Verification items for the finished model (mm, model axes). Face numbers are marked on the shaded views. A direction names the side the tool comes from. Coordinates: 2 decimals unless noted, no trailing zeros. Order: outer loops, then holes, each group sorted by start corner. A loop starts at its lowest first (then second) coordinate and runs counter-clockwise, first axis right, second up. Notation, with made-up numbers: (-24, 21) -> (8, 21) arc R18 cw to (8, 46) -> close; hole circle Ø10 at (0.5, 63.5). An arc over 180 degrees is marked (long way). Use CSV: the item, a comma, the result in double quotes. Start each with the question number.
1) Tool access check on the marked faces 1, 2 and 3. Record the directions out of +Z, -Z, +X, -X, +Y, -Y that give a thin tool (end or side, any length) a straight path to the whole face; none if there is none.
2) Go/stop test with flat-tipped pins: pin 1 (8.5 mm diameter, centred on x = 0, y = -8, fed in from +Z); pin 2 (8.5 mm diameter, centred on x = 0, y = -8, fed in from -Z); pin 3 (2.5 mm diameter, centred on x = 11.5, z = 1, fed in from +Y); pin 4 (5.5 mm diameter, centred on x = 11.25, y = -5.25, fed in from -Z). Record where each tip stops, or that it passes through.
3) Scan lines: line 1 along Y through (x, z) = (1.5, 1.6) (3 decimals); line 2 along Y through (x, z) = (0, 4.2); line 3 along X through (y, z) = (6.5, 3.7). Record each from-to range of solid material in increasing order.
4) Sectioned sample at D-D on y = -7.5. Record the boundary of the cut face in (x, z), then the cut area to 3 significant figures.
5) Sectioned sample at A-A on x = 0. Record the boundary of the cut face in (y, z), then the cut area to 3 significant figures.
6) Sectioned sample at B-B on x = -11.25. Record the boundary of the cut face in (y, z), then the cut area to 3 significant figures.
7) Release check for a two-part mould opening along Y. For the marked faces 4, 5 and 6 record: released by +Y, released by -Y, zero draft, split by the parting line, or undercut.
8) Sectioned sample at C-C on z = 3.8. Give the number of separate pieces and of enclosed holes in the cut face, then the cut area to 3 significant figures.
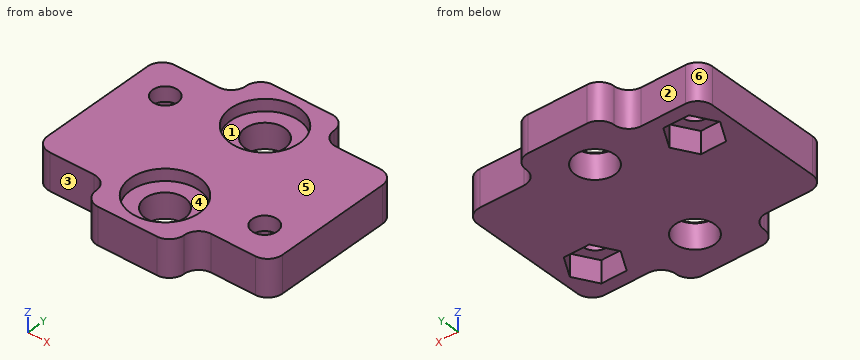
from build123d import *

# Parameters (mm, degrees)
SCHIZZO1_W                   = 32
SCHIZZO1_H                   = 20
ESTRUSIONE_ESTRUSIONE1_DEPTH = 5
SCHIZZO2_R                   = 1.7
TAGLIO_ESTRUSIONE1_DEPTH     = 20.519221296
SCHIZZO3_W                   = 12
SCHIZZO3_H                   = 4
ESTRUSIONE_ESTRUSIONE2_DEPTH = 5
SCHIZZO4_R                   = 4.7
TAGLIO_ESTRUSIONE2_DEPTH     = 1.6
SCHIZZO5_R                   = 2.7
TAGLIO_ESTRUSIONE3_DEPTH     = 22.530443563
TAGLIO_ESTRUSIONE4_DEPTH     = 3
RACCORDO1_R                  = 2


with BuildPart() as part:
    # Schizzo1 → Estrusione-Estrusione1 (new body)
    with BuildSketch(Plane.XY):
        Rectangle(SCHIZZO1_W, SCHIZZO1_H)
    extrude(amount=ESTRUSIONE_ESTRUSIONE1_DEPTH)

    # Schizzo2 → Taglio-Estrusione1 (cut, through all)
    with BuildSketch(Plane.XY.offset(5)):
        with Locations((-11.25, 5.25)):
            Circle(SCHIZZO2_R)
        with Locations((11.25, -5.25)):
            Circle(SCHIZZO2_R)
    extrude(amount=-TAGLIO_ESTRUSIONE1_DEPTH, mode=Mode.SUBTRACT)

    # Schizzo3 → Estrusione-Estrusione2 (add)
    with BuildSketch(Plane.XY):
        with Locations((0, 12)):
            Rectangle(SCHIZZO3_W, SCHIZZO3_H)
        with Locations((0, -12)):
            Rectangle(SCHIZZO3_W, SCHIZZO3_H)
    extrude(amount=ESTRUSIONE_ESTRUSIONE2_DEPTH)

    # Schizzo4 → Taglio-Estrusione2 (cut)
    with BuildSketch(Plane.XY.offset(5)):
        with Locations((0, 8)):
            Circle(SCHIZZO4_R)
        with Locations(Location((0, -8, 0), (0, 0, 180))):
            Circle(SCHIZZO4_R)
    extrude(amount=-TAGLIO_ESTRUSIONE2_DEPTH, mode=Mode.SUBTRACT)

    # Schizzo5 → Taglio-Estrusione3 (cut, through all)
    with BuildSketch(Plane.XY.offset(3.4)):
        with Locations((0, 8)):
            Circle(SCHIZZO5_R)
        with Locations((0, -8)):
            Circle(SCHIZZO5_R)
    extrude(amount=-TAGLIO_ESTRUSIONE3_DEPTH, mode=Mode.SUBTRACT)

    # Schizzo6 → Taglio-Estrusione4 (cut)
    with BuildSketch(Plane(origin=(0, 0, 0), x_dir=(-1, 0, 0), z_dir=(0, 0, -1))):
        Polygon((7.785898385, 5.25), (9.517949192, 2.25), (12.982050808, 2.25), (14.714101615, 5.25), (12.982050808, 8.25), (9.517949192, 8.25), align=None)
        Polygon((-14.714101615, -5.25), (-12.982050808, -8.25), (-9.517949192, -8.25), (-7.785898385, -5.25), (-9.517949192, -2.25), (-12.982050808, -2.25), align=None)
    extrude(amount=-TAGLIO_ESTRUSIONE4_DEPTH, mode=Mode.SUBTRACT)

    # Raccordo1
    raccordo1_edges = [part.edges().sort_by_distance(p)[0] for p in [
        (16, 10, 2.5),
        (16, -10, 2.5),
        (6, -10, 2.5),
        (6, -14, 2.5),
        (-6, -14, 2.5),
        (-6, -10, 2.5),
        (-16, -10, 2.5),
        (-16, 10, 2.5),
        (6, 14, 2.5),
        (-6, 14, 2.5),
        (-6, 10, 2.5),
        (6, 10, 2.5),
    ]]
    fillet(raccordo1_edges, radius=RACCORDO1_R - 0.0001)  # a hair under: the kernel refuses the full size


solid = part.part
Answers follow:
1,face 1,"+Z"
1,face 2,"+Z, -Z, -X, +Y"
1,face 3,"+Z, -Z, -X, -Y"
2,pin 1,"stops at z = 3.4"
2,pin 2,"stops at z = 0"
2,pin 3,"stops at y = 10"
2,pin 4,"stops at z = 3"
3,line 1,"y = -14 to -10.245, -5.755 to 5.755, 10.245 to 14"
3,line 2,"y = -14 to -12.7, -3.3 to 3.3, 12.7 to 14"
3,line 3,"x = -16 to -12.4, -10.1 to -4.45, 4.45 to 16"
4,outline,"(-16, 0) -> (-2.65, 0) -> (-2.65, 3.4) -> (-4.67, 3.4) -> (-4.67, 5) -> (-16, 5) -> close; (2.65, 0) -> (9.08, 0) -> (9.08, 3) -> (13.42, 3) -> (13.42, 0) -> (16, 0) -> (16, 5) -> (4.67, 5) -> (4.67, 3.4) -> (2.65, 3.4) -> close"
4,area,"114 mm²"
5,outline,"(-14, 0) -> (-10.7, 0) -> (-10.7, 3.4) -> (-12.7, 3.4) -> (-12.7, 5) -> (-14, 5) -> close; (-5.3, 0) -> (5.3, 0) -> (5.3, 3.4) -> (3.3, 3.4) -> (3.3, 5) -> (-3.3, 5) -> (-3.3, 3.4) -> (-5.3, 3.4) -> close; (10.7, 0) -> (14, 0) -> (14, 5) -> (12.7, 5) -> (12.7, 3.4) -> (10.7, 3.4) -> close"
5,area,"73.2 mm²"
6,outline,"(-10, 0) -> (2.25, 0) -> (2.25, 3) -> (3.55, 3) -> (3.55, 5) -> (-10, 5) -> close; (6.95, 3) -> (8.25, 3) -> (8.25, 0) -> (10, 0) -> (10, 5) -> (6.95, 5) -> close"
6,area,"75.2 mm²"
7,face 4,"undercut"
7,face 5,"zero draft"
7,face 6,"released by +Y"
8,separate pieces,"1"
8,enclosed holes,"4"
8,area,"576 mm²"
